```python
from build123d import *

# Parameters (mm, degrees)
F1_DEPTH  = 21
F3_DEPTH  = 4.3
F4_R      = 2.625
F5_DEPTH  = 27.677358
F6_R      = 4.125
F7_DEPTH  = 4.15
F9_R      = 4
F10_DEPTH = 3.1
F11_R     = 2.63
F12_DEPTH = 15.4
F13_R     = 2.194009
F13_R_2   = 2.575
F13_R_3   = 1.491787
F14_DEPTH = 18.4


with BuildPart() as f1:
    # F0 (on Top) → F1 (new body)
    with BuildSketch(Plane.XY):
        with BuildLine():
            ThreePointArc((-10.851728, 1.8), (11, 0), (-10.851728, -1.8))
            Line((-10.851728, -1.8), (-15.697133, -1.8))
            ThreePointArc((-15.697133, -1.8), (-14.879747, -5.313485), (-13.286742, -8.55))
            ThreePointArc((-13.286742, -8.55), (-5.672485, -14.746624), (4.131669, -15.250223))
            ThreePointArc((4.131669, -15.250223), (7.383686, -15.469855), (9.809368, -17.646991))
            Line((9.809368, -17.646991), (10.735537, -19.313162))
            ThreePointArc((10.735537, -19.313162), (16.894368, -23.382819), (23.762893, -20.677885))
            ThreePointArc((23.762893, -20.677885), (31.5, 0), (23.762893, 20.677885))
            ThreePointArc((23.762893, 20.677885), (16.894368, 23.382819), (10.735537, 19.313162))
            Line((10.735537, 19.313162), (9.809368, 17.646991))
            ThreePointArc((9.809368, 17.646991), (7.383686, 15.469855), (4.131669, 15.250223))
            ThreePointArc((4.131669, 15.250223), (-5.672485, 14.746624), (-13.286742, 8.55))
            ThreePointArc((-13.286742, 8.55), (-14.879747, 5.313485), (-15.697133, 1.8))
            Line((-15.697133, 1.8), (-10.851728, 1.8))
        make_face()
        Polygon((14.5, -16), (14.5, 0), (14.5, 16), (19.5, 16), (19.5, -16), align=None, mode=Mode.SUBTRACT)
        with BuildLine():
            ThreePointArc((-13.286742, -8.55), (-14.879747, -5.313485), (-15.697133, -1.8))
            Line((-15.697133, -1.8), (-30.5, -1.8))
            ThreePointArc((-30.5, -1.8), (-31.207107, -2.092893), (-31.5, -2.8))
            Line((-31.5, -2.8), (-31.5, -5.55))
            ThreePointArc((-31.5, -5.55), (-30.62132, -7.67132), (-28.5, -8.55))
            Line((-28.5, -8.55), (-13.286742, -8.55))
        make_face()
        with BuildLine():
            Line((-30.5, 1.8), (-15.697133, 1.8))
            ThreePointArc((-15.697133, 1.8), (-14.879747, 5.313485), (-13.286742, 8.55))
            Line((-13.286742, 8.55), (-28.5, 8.55))
            ThreePointArc((-28.5, 8.55), (-30.62132, 7.67132), (-31.5, 5.55))
            Line((-31.5, 5.55), (-31.5, 2.8))
            ThreePointArc((-31.5, 2.8), (-31.207107, 2.092893), (-30.5, 1.8))
        make_face()
    extrude(amount=F1_DEPTH)

    # F2 (on face) → F3 (cut)
    with BuildSketch(Plane.XZ.offset(8.55)):
        Polygon((-23.268371, 14.613621), (-25.643371, 10.5), (-23.268371, 6.386379), (-18.518371, 6.386379), (-16.143371, 10.5), (-18.518371, 14.613621), align=None)
    extrude(amount=-F3_DEPTH, mode=Mode.SUBTRACT)

    # F4 (on face) → F5 (cut, through all)
    with BuildSketch(Plane.XZ.offset(4.25)):
        with Locations((-20.893371, 10.5)):
            Circle(F4_R)
    extrude(amount=-F5_DEPTH, mode=Mode.SUBTRACT)

    # F6 (on face) → F7 (cut)
    with BuildSketch(Plane(origin=(0, 8.55, 0), x_dir=(-1, 0, 0), z_dir=(0, 1, 0))):
        with Locations((20.893371, 10.5)):
            Circle(F6_R)
    extrude(amount=-F7_DEPTH, mode=Mode.SUBTRACT)

    # F9 (on offset) → F10 (cut)
    with BuildSketch(Plane.YZ.offset(31.5)):
        with Locations((0, 10.5)):
            Circle(F9_R)
    extrude(amount=-F10_DEPTH, mode=Mode.SUBTRACT)

    # F11 (on face) → F12 (cut)
    with BuildSketch(Plane.YZ.offset(28.4)):
        with Locations((0, 10.5)):
            Circle(F11_R)
    extrude(amount=-F12_DEPTH, mode=Mode.SUBTRACT)

    # F13 (on face) → F14 (cut)
    with BuildSketch(Plane(origin=(0, 0, 0), x_dir=(1, 0, 0), z_dir=(0, 0, -1))):
        with Locations((10.025991, 11.786622)):
            Circle(F13_R)
        with Locations((10.025991, -11.786622)):
            Circle(F13_R)
        with Locations((24.775, 7.968689)):
            Circle(F13_R_2)
        with Locations((24.775, -7.968689)):
            Circle(F13_R_2)
        with Locations((16.947184, 19.69141)):
            Circle(F13_R_3)
        with Locations((16.947184, -19.69141)):
            Circle(F13_R_3)
    extrude(amount=-F14_DEPTH, mode=Mode.SUBTRACT)


solid = f1.part
```
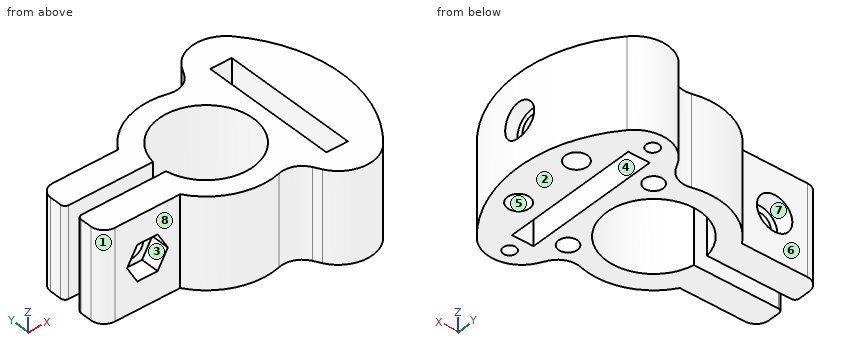
Geometry: final body of the model. Coordinates: model frame, mm. Face numbers are marked on the shaded views. A direction names the side the tool comes from. Round coordinates to 2 decimals unless told otherwise and drop trailing zeros. Order: outer loops, then holes, each group sorted by start corner. A loop starts at its lowest first (then second) coordinate and runs counter-clockwise, first axis right, second up. Notation, with made-up numbers: (-30.5, 8) - (21.5, 8) arc R23 ccw to (21.5, 37) - close; hole circle Ø1 at (84.25, 35.5). An arc over 180 degrees is marked (long way). Write item = value, one per line. Start each with the question number.
Q1. Ray query, line 1 (Y direction, x = 8.5, z = 12.75); line 2 (Y direction, x = -21, z = 7); line 3 (Y direction, x = -25.5, z = 19.25). Return the intervals inside material, ascending. Write a range as from..to.
Q2. Cut plane C-C on x = 0. Return the cut outline in (y, z), and give its area (3 significant figures).
Q3. Cut plane B-B on x = -14.5. Return the cut outline in (y, z).
Q4. Pin query (flat end, axial travel): pin 1 (4 mm diameter, centred on x = 24.78, y = 7.97, fed in from -Z); pin 2 (8 mm diameter, centred on x = -17.5, z = 16, fed in from +Y); pin 3 (8 mm diameter, centred on x = 11.5, z = 9, fed in from -Y); pin 4 (1 mm diameter, centred on x = 16.5, y = -8.5, fed in from -Z). Return the tip coordinate at first contact, or that it passes through.
Q5. Access query for the marked faces 5, 6, 7 and 8. Directions: +Z, -Z, +X, -X, +Y, -Y. A direction counts if a zero-diameter tool reaches every point of the face in a straight line with its end or side. Return the directions, or none.
Q6. Cut plane D-D on z = 3. Give the number of separate pieces and of enclosed holes in the cut face, and give its area (3 significant figures).
Q7. Pull-direction query (X, two-part tool) for the marked faces 1, 2, 3 and 4; classes: +X half, -X half, draft (parallel to the pull), parting line (faces both ways), or undercut.
Q8. Cut plane A-A on y = 0. Return the cut outline in (x, z), and give its area (3 significant figures).
Outcome:
q1.line_1 = -16.12..-13.36, -10.21..-6.98, 6.98..10.21, 13.36..16.12
q1.line_2 = -4.25..-1.8, 1.8..4.4
q1.line_3 = -8.55..-1.8, 1.8..8.55
q2.outline = (-15.8, 0) - (-11, 0) - (-11, 21) - (-15.8, 21) - close; (11, 0) - (15.8, 0) - (15.8, 21) - (11, 21) - close
q2.area = 202 mm^2
q3.outline = (-8.55, 0) - (-1.8, 0) - (-1.8, 21) - (-8.55, 21) - close; (1.8, 0) - (8.55, 0) - (8.55, 21) - (1.8, 21) - close
q4.pin_1 = 18.4
q4.pin_2 = 8.55
q4.pin_3 = -23.11
q4.pin_4 = through
q5.face_5 = -Z
q5.face_6 = +Z, -Z, -X, +Y
q5.face_7 = +Y
q5.face_8 = +Z, -Z, -X, -Y
q6.separate_pieces = 1
q6.enclosed_holes = 7
q6.area = 1,110 mm^2
q7.face_1 = -X half
q7.face_2 = draft
q7.face_3 = undercut
q7.face_4 = undercut
q8.outline = (11, 0) - (14.5, 0) - (14.5, 7.87) - (13, 7.87) - (13, 13.13) - (14.5, 13.13) - (14.5, 21) - (11, 21) - close; (19.5, 0) - (31.5, 0) - (31.5, 6.5) - (28.4, 6.5) - (28.4, 7.87) - (19.5, 7.87) - close; (19.5, 13.13) - (28.4, 13.13) - (28.4, 14.5) - (31.5, 14.5) - (31.5, 21) - (19.5, 21) - close
q8.area = 246 mm^2
